```python
from build123d import *

# Parameters (mm, degrees)
BOSS_EXTRUDE1_DEPTH          = 3.175
CHAMFER1_SIZE                = 6.35
FILLET1_R                    = 12.7
F_3_8_0_375_DIAMETER_HOLE1_D = 9.525
F_8_CLEARANCE_HOLE1_D        = 4.064
FILLET2_R                    = 3.175
FILLET3_R                    = 3.175
F_8_CLEARANCE_HOLE2_D        = 4.064


with BuildPart() as part:
    # Sketch1 → Boss-Extrude1 (new body)
    with BuildSketch(Plane(origin=(0, 0, 0), x_dir=(0, 0, -1), z_dir=(1, 0, 0))):
        with BuildLine():
            Line((-184.15, -24.60625), (184.15, -24.60625))
            Line((184.15, -24.60625), (184.15, 26.19375))
            Line((184.15, 26.19375), (146.05, 26.19375))
            Line((146.05, 26.19375), (57.15, 280.19375))
            Line((57.15, 280.19375), (-69.85, 305.59375))
            Line((-69.85, 305.59375), (-103.309941035, 336.853985858))
            ThreePointArc((-103.309941035, 336.853985858), (-129.244818111, 342.195404789), (-145.838997174, 321.560923299))
            Line((-145.838997174, 321.560923299), (-184.15, 26.19375))
            Line((-184.15, 26.19375), (-184.15, -24.60625))
        make_face()
    extrude(amount=BOSS_EXTRUDE1_DEPTH)

    # Chamfer1
    chamfer1_edges = [part.edges().sort_by_distance(p)[0] for p in [
        (1.5875, -24.60625, -184.15),
        (1.5875, -24.60625, 184.15),
    ]]
    chamfer(chamfer1_edges, length=CHAMFER1_SIZE)

    # Fillet1
    fillet1_edges = [part.edges().sort_by_distance(p)[0] for p in [
        (1.5875, 305.59375, 69.85),
        (1.5875, 280.19375, -57.15),
    ]]
    fillet(fillet1_edges, radius=FILLET1_R)

    # 3/8 (0.375) Diameter Hole1 (through all)
    with Locations(Plane.ZY):
        with Locations((-112.174577673, 0.79375), (-74.074577673, 0.79375), (-35.974577673, 0.79375), (35.974577673, 0.79375), (74.074577673, 0.79375)):
            Hole(F_3_8_0_375_DIAMETER_HOLE1_D / 2)

    # #8 Clearance Hole1 (through all)
    with Locations(Plane.ZY):
        with Locations((148.157911006, 0.79375), (112.174577673, 0.79375), (-148.157911006, 0.79375), (0, 0)):
            Hole(F_8_CLEARANCE_HOLE1_D / 2)

    # Fillet2
    fillet2_edges = [part.edges().sort_by_distance(p)[0] for p in [
        (1.5875, 26.19375, 184.15),
        (1.5875, 26.19375, -146.05),
        (1.5875, 26.19375, -184.15),
    ]]
    fillet(fillet2_edges, radius=FILLET2_R)

    # Fillet3
    fillet3_edges = [part.edges().sort_by_distance(p)[0] for p in [
        (1.5875, -24.60625, -177.8),
        (1.5875, -24.60625, 177.8),
        (1.5875, -18.25625, 184.15),
        (1.5875, -18.25625, -184.15),
    ]]
    fillet(fillet3_edges, radius=FILLET3_R)

    # #8 Clearance Hole2 (through all)
    with Locations(Plane(origin=(3.175, 0, 0), x_dir=(0, 0, -1), z_dir=(1, 0, 0))):
        with Locations((-179.705, 21.74875), (-179.705, -16.415070715), (179.705, 21.74875), (179.3875, -16.283557909)):
            Hole(F_8_CLEARANCE_HOLE2_D / 2)


solid = part.part
```
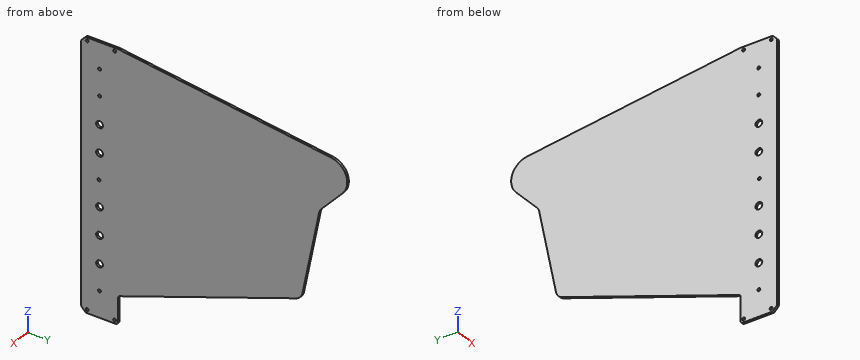
Here's how the part is built. I have some questions about the finished solid (model axes, mm). Round coordinates to 2 decimals unless told otherwise and drop trailing zeros. Loops run counter-clockwise (first coordinate to the right, second up) from the corner with the lowest first, then second, coordinate; pieces in that order, holes last.
1. Suppose I cut it at C-C, the plane y = 74. Please give me the cut outline in (x, z) (3 decimals), and give its area (3 significant figures).
Answers:
outline: (0, -129.318) - (3.175, -129.318) - (3.175, 177.949) - (0, 177.949) - close
area: 976 mm2
2. If I drill on probe 1 along Y at (x, z) = (1.15, 0); probe 2 along Z at (x, y) = (2, 191); probe 3 along Z at (x, y) = (2, 171), over which ranges is the centre line in solid material (lowest first)?
Answers:
probe 1: y = -24.61 to -2.03, 2.03 to 291.62
probe 2: z = -88.37 to 162.77
probe 3: z = -95.37 to 165.37
3. Will these pins go through, and if not, where does the flat tip stop? pin 1 (1.5 mm diameter, centred on x = 2, z = 3.5, fed in from +Y); pin 2 (1.6 mm diameter, centred on x = 1.5, z = -158.5, fed in from +Y); pin 3 (1 mm diameter, centred on x = 2.5, z = 132, fed in from +Y).
Answers:
pin 1: stops at y = 292.47
pin 2: stops at y = 26.19
pin 3: stops at y = 341.26
4. Suppose I cut it at B-B, the plane z = -160.5. Please give me the cut outline in (x, y) (3 decimals).
Answers:
outline: (0, -24.606) - (3.175, -24.606) - (3.175, 26.194) - (0, 26.194) - close
5. Suppose I cut it at A-A, the plane x = 1.05. Give the number of separate pieces and of enclosed holes in the cut face, and give its area (3 significant figures).
Answers:
separate pieces: 1
enclosed holes: 13
area: 92,200 mm2
